```python
from build123d import *

# Parameters (mm, degrees)
SKETCH1_W           = 5
SKETCH1_H           = 5
BOSS_EXTRUDE1_DEPTH = 127.3
SKETCH2_W           = 2.5
SKETCH2_H           = 2.5
BOSS_EXTRUDE2_DEPTH = 5
SKETCH3_W           = 2.5
SKETCH3_H           = 2.5
BOSS_EXTRUDE3_DEPTH = 5
SKETCH4_W           = 3
SKETCH4_H           = 3
CUT_EXTRUDE1_DEPTH  = 30
SKETCH7_W           = 127.3
SKETCH7_H           = 1.5
CUT_EXTRUDE5_DEPTH  = 2


with BuildPart() as part:
    # Sketch1 → Boss-Extrude1 (new body)
    with BuildSketch(Plane.XY):
        with Locations((2.5, 2.5)):
            Rectangle(SKETCH1_W, SKETCH1_H)
    extrude(amount=BOSS_EXTRUDE1_DEPTH)

    # Sketch2 → Boss-Extrude2 (add)
    with BuildSketch(Plane(origin=(0, 0, 0), x_dir=(-1, 0, 0), z_dir=(0, 0, -1))):
        with Locations((-2.5, 2.5)):
            Rectangle(SKETCH2_W, SKETCH2_H)
    extrude(amount=BOSS_EXTRUDE2_DEPTH)

    # Sketch3 → Boss-Extrude3 (add)
    with BuildSketch(Plane.XY.offset(127.3)):
        with Locations((2.5, 2.5)):
            Rectangle(SKETCH3_W, SKETCH3_H)
    extrude(amount=BOSS_EXTRUDE3_DEPTH)

    # Sketch4 → Cut-Extrude1 (cut)
    with BuildSketch(Plane.ZY):
        with Locations((120.8, 2.5)):
            Rectangle(SKETCH4_W, SKETCH4_H)
        with Locations((51.5, 2.5)):
            Rectangle(SKETCH4_W, SKETCH4_H)
        with Locations((72.8, 2.5)):
            Rectangle(SKETCH4_W, SKETCH4_H)
    extrude(amount=-CUT_EXTRUDE1_DEPTH, mode=Mode.SUBTRACT)

    # Sketch7 → Cut-Extrude5 (cut)
    with BuildSketch(Plane(origin=(5, 0, 0), x_dir=(0, 0, -1), z_dir=(1, 0, 0))):
        with Locations((-63.65, 2.5)):
            Rectangle(SKETCH7_W, SKETCH7_H)
    extrude(amount=-CUT_EXTRUDE5_DEPTH, mode=Mode.SUBTRACT)


solid = part.part
```
Input: part model. Units: mm. Frame: model coordinates. A direction names the side the tool comes from. Give positions to 0.01 mm unless a question says otherwise; leave off trailing zeros. Order: outer loops, then holes, each group sorted by start corner. A loop starts at its lowest first (then second) coordinate and runs counter-clockwise, first axis right, second up.
1. Pin query (flat end, axial travel): pin 1 Ø0.6 at (x, z) = (4, 126) entering from -Y; pin 2 Ø2 at (y, z) = (3, -1.5) entering from -X; pin 3 Ø3 at (x, z) = (2.5, 129.5) entering from -Y; pin 4 Ø3 at (y, z) = (3, 130.5) entering from +X. Return the tip coordinate at first contact, or that it passes through.
Computed:
pin 1: stops at y = 0
pin 2: stops at x = 1.25
pin 3: stops at y = 1.25
pin 4: stops at x = 3.75
2. Set-up query: faces 1 (the face through (1.25, 2, -2)), 2 (the face through (3.75, 2, 130)), 3 (the face through (1.25, 2, 130)), 4 (the face through (2, 1.25, 130)). Return all of +Z, -Z, +X, -X, +Y, -Y with unobstructed straight access to the full face (end or side cutting, diameter ignored); none if empty.
Computed:
face 1: -Z, -X, +Y, -Y
face 2: +Z, +X, +Y, -Y
face 3: +Z, -X, +Y, -Y
face 4: +Z, +X, -X, -Y
3. Cut plane A-A (x = 2). Return loops of the section in (y, z).
Computed:
outline: (0, 0) - (1.25, 0) - (1.25, -5) - (3.75, -5) - (3.75, 0) - (5, 0) - (5, 127.3) - (3.75, 127.3) - (3.75, 132.3) - (1.25, 132.3) - (1.25, 127.3) - (0, 127.3) - close; hole (1, 50) - (4, 50) - (4, 53) - (1, 53) - close; hole (1, 71.3) - (4, 71.3) - (4, 74.3) - (1, 74.3) - close; hole (1, 119.3) - (4, 119.3) - (4, 122.3) - (1, 122.3) - close
4. Line query: probe 1 along Z at (x, y) = (4.8, 3.55); probe 2 along Z at (x, y) = (1.85, 3.6); probe 3 along Y at (x, z) = (3.1, 60). Output: solid intervals per line, ascending.
Computed:
probe 1: z = 0 to 50, 53 to 71.3, 74.3 to 119.3, 122.3 to 127.3
probe 2: z = -5 to 50, 53 to 71.3, 74.3 to 119.3, 122.3 to 132.3
probe 3: y = 0 to 1.75, 3.25 to 5
5. Cut plane B-B (z = 30). Return loops of the section in (x, y), and give its area (3 significant figures).
Computed:
outline: (0, 0) - (5, 0) - (5, 1.75) - (3, 1.75) - (3, 3.25) - (5, 3.25) - (5, 5) - (0, 5) - close
area: 22.0 mm2
